Geometry: see drawing. Coordinates: mm, zero at the bounding-box minimum. A direction names the side the tool comes from. Round coordinates to 2 decimals unless told otherwise and drop trailing zeros. Order: outer loops, then holes, each group sorted by start corner. A loop starts at its lowest first (then second) coordinate and runs counter-clockwise, first axis right, second up. Notation, with made-up numbers: (-16, -26) -> (6, -26) arc R10 ccw to (6, -15) -> close; hole circle Ø8 at (13, 69). An arc over 180 degrees is marked (long way). Use a Markdown table: item, result.
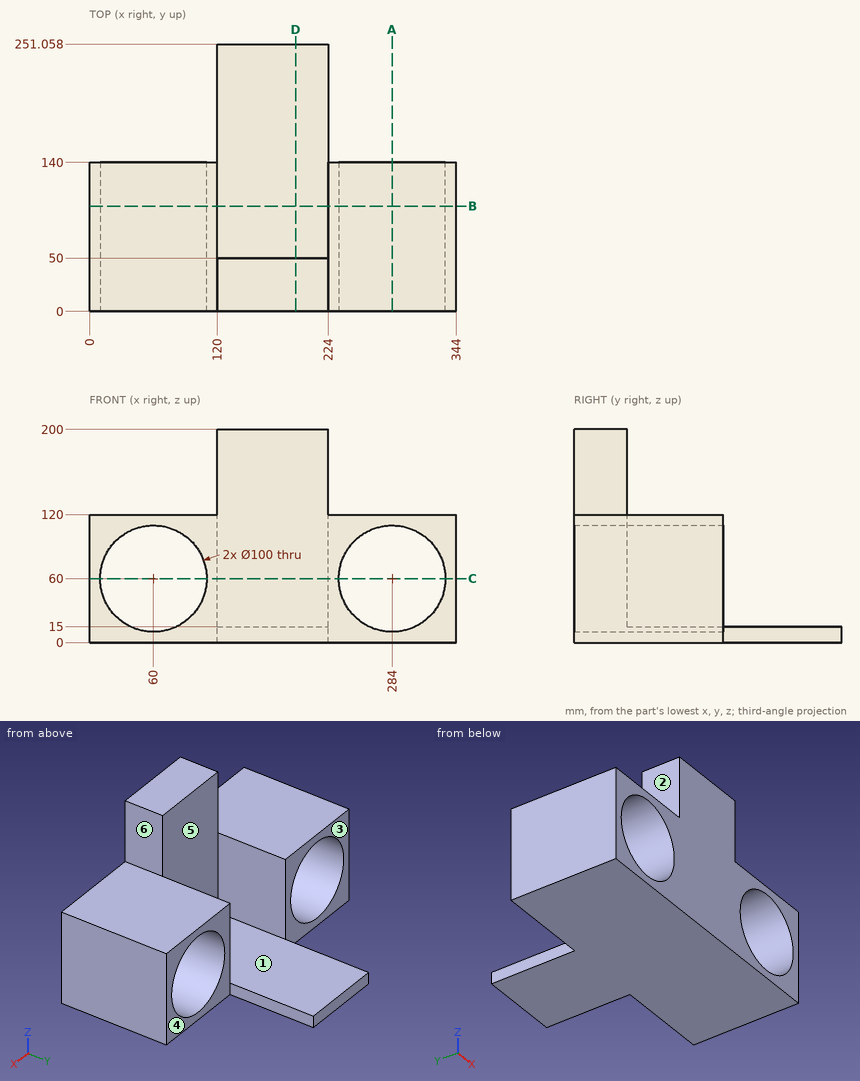
1) Cut plane D-D on x = 193.5. Return loops of the section in (y, z).
Answer key:
| item | result |
|---|---|
| outline | (0, 0) -> (251.06, 0) -> (251.06, 15) -> (50, 15) -> (50, 200) -> (0, 200) -> close |
2) Set-up query: the marked faces 4, 5 and 6. Return all of +Z, -Z, +X, -X, +Y, -Y with unobstructed straight access to the full face (end or side cutting, diameter ignored); none if empty.
Answer key:
| item | result |
|---|---|
| face 4 | +Z, -Z, +X, +Y |
| face 5 | +Z, +Y |
| face 6 | +Z, +X, +Y, -Y |
3) Cut plane A-A on x = 284. Return loops of the section in (y, z), and give its area (3 significant figures).
Answer key:
| item | result |
|---|---|
| outline | (0, 0) -> (140, 0) -> (140, 10) -> (0, 10) -> close; (0, 110) -> (140, 110) -> (140, 120) -> (0, 120) -> close |
| area | 2,800 mm^2 |
4) Cut plane C-C on z = 60. Return loops of the section in (x, y).
Answer key:
| item | result |
|---|---|
| outline | (0, 0) -> (10, 0) -> (10, 140) -> (0, 140) -> close; (110, 0) -> (234, 0) -> (234, 140) -> (224, 140) -> (224, 50) -> (120, 50) -> (120, 140) -> (110, 140) -> close; (334, 0) -> (344, 0) -> (344, 140) -> (334, 140) -> close |
5) Draft query along X for the marked faces 1, 2 and 3. Return one class per face: released by +X, released by -X, zero draft, split by the parting line, or undercut.
Answer key:
| item | result |
|---|---|
| face 1 | undercut |
| face 2 | released by -X |
| face 3 | zero draft |
6) Contact query for flat-ended pins moving along their axis: P1, Ø7.5, axis at y = 190, z = 9.5, coming from the -X side; P2, Ø16.5, axis at y = 171, z = 7, coming from the +X side; P3, Ø1.5, axis at x = 130, y = 130.5, coming from the -Z side. Output: stop coordinate, or through.
Answer key:
| item | result |
|---|---|
| P1 | stops at x = 120 |
| P2 | stops at x = 224 |
| P3 | stops at z = 0 |
7) Cut plane B-B on y = 99. Return loops of the section in (x, z), and give its area (3 significant figures).
Answer key:
| item | result |
|---|---|
| outline | (0, 0) -> (344, 0) -> (344, 120) -> (224, 120) -> (224, 15) -> (120, 15) -> (120, 120) -> (0, 120) -> close; hole circle Ø100 at (60, 60); hole circle Ø100 at (284, 60) |
| area | 14,700 mm^2 |
8) Ray query, probe 1 along X at (y, z) = (128, 61); probe 2 along Z at (x, y) = (60, 101); probe 3 along Y at (x, z) = (281, 119.5). Return the intervals inside material, ascending.
Answer key:
| item | result |
|---|---|
| probe 1 | x = 0 to 10.01, 109.99 to 120, 224 to 234.01, 333.99 to 344 |
| probe 2 | z = 0 to 10, 110 to 120 |
| probe 3 | y = 0 to 140 |
